Read the model definition and answer for the solid it produces. Units are mm, in the model's axes. A direction names the side the tool comes from. Give positions to 0.01 mm unless a question says otherwise; leave off trailing zeros. Loops run counter-clockwise (first coordinate to the right, second up) from the corner with the lowest first, then second, coordinate; pieces in that order, holes last. Notation, with made-up numbers: (60.5, 70) - (115.5, 70) arc R7 cw to (115.5, 82) - close; hole circle Ø11 at (-40, 17.5). An arc over 180 degrees is marked (long way). Write each question's results on one line, items separated by ' | '. Start each with the question number.
Q1. The part is cut by section B-B, the plane z = 0. Write down the section's boundary in (x, y).
Q2. Given pin 1 (3 mm diameter, centred on y = 5.5, z = 6, fed in from -X); pin 2 (2 mm diameter, centred on y = 13.5, z = -4.5, fed in from -X); pin 3 (4 mm diameter, centred on x = -31, y = 5.5, fed in from -Z), each flat-ended and moving along its own axis, determine where each tip first touches the part or whether it passes through.
Q3. The part is cut by section D-D, the plane x = -7.5. Write down the section's boundary in (y, z).
Q4. Find the intervals of material crossed by line 1 (X direction, y = 6, z = -6.75); line 2 (Z direction, x = -14.5, y = 2.75); line 3 (Y direction, x = -14, z = 1), in increasing order. Write a range as from..to.
Q5. For faces 1 (the flat face through (14, 17, 0)), 2 (the cylindrical face through (5.997, 13.451, -1.843)), determine the directions among +Z, -Z, +X, -X, +Y, -Y from which every point of the face is accessible in a straight line to the end or side of a thin tool.
Q6. The part is cut by section C-C, the plane y = 6.25. Write down the section's boundary in (x, z).
Q7. Determine the mould class of faces 3 (the cylindrical face through (-19.431, 4.93, 8.134)), 4 (the flat face through (-25, 5, 3)), 5 (the cylindrical face through (-35.35, 2.26, -0.61)) for opening direction Z: +Z half, -Z half, draft (parallel to the pull), parting line (faces both ways), or undercut.
Q8. The part is cut by section A-A, the plane z = 4.5. Write down the section's boundary in (x, y).
```python
from build123d import *

# Parameters (mm, degrees)
SKETCH_1_W      = 50
SKETCH_1_H      = 25
SKETCH_1_R      = 8.5
SKETCH_1_R_2    = 3
EXTRUDE_1_DEPTH = 10
SKETCH_2_R      = 2.808756841
EXTRUDE_2_DEPTH = 21
SKETCH_1_3_R    = 8.5
EXTRUDE_3_DEPTH = 17


with BuildPart() as part:
    # Sketch 1 → Extrude 1 (new body)
    # profile 1 of 2: a face of its own
    with BuildSketch(Plane(origin=(0, 0, 0), x_dir=(1, 0, 0), z_dir=(0, 1, 0))):
        Rectangle(SKETCH_1_W, SKETCH_1_H)
        with Locations((14.294554455, 0)):
            Circle(SKETCH_1_R, mode=Mode.SUBTRACT)
        with Locations(Location((-16.76980198, 6.75, 0), (0, 0, 270))):
            Circle(SKETCH_1_R_2, mode=Mode.SUBTRACT)
        with Locations(Location((-16.76980198, -6.75, 0), (0, 0, 270))):
            Circle(SKETCH_1_R_2, mode=Mode.SUBTRACT)
    # profile 2 of 2: a face of its own
    with BuildSketch(Plane(origin=(0, 0, 0), x_dir=(1, 0, 0), z_dir=(0, 1, 0))):
        with Locations((14.294554455, 0)):
            Circle(SKETCH_1_R)
    extrude(amount=EXTRUDE_1_DEPTH)

    # Sketch 2 → Extrude 2 (add)
    with BuildSketch(Plane.ZY.offset(25)):
        with Locations((0, 5)):
            Circle(SKETCH_2_R)
    extrude(amount=EXTRUDE_2_DEPTH)

    # Sketch 1_3 → Extrude 3 (add)
    with BuildSketch(Plane(origin=(0, 0, 0), x_dir=(1, 0, 0), z_dir=(0, 1, 0))):
        with Locations(Location((14.294554455, 0, 0), (0, 0, 270))):
            Circle(SKETCH_1_3_R)
    extrude(amount=EXTRUDE_3_DEPTH)


solid = part.part
```
Check sheet entries:
1) outline: (-46, 2.19) - (-25, 2.19) - (-25, 0) - (25, 0) - (25, 10) - (22.79, 10) - (22.79, 17) - (5.79, 17) - (5.79, 10) - (-25, 10) - (-25, 7.81) - (-46, 7.81) - close
2) pin 1: stops at x = -25 | pin 2: stops at x = 6.55 | pin 3: stops at z = -2.81
3) outline: (0, -12.5) - (10, -12.5) - (10, 12.5) - (0, 12.5) - close
4) line 1: x = -25..-19.77, -13.77..25 | line 2: z = -12.5..-8.71, -4.79..4.79, 8.71..12.5 | line 3: y = 0..10
5) face 1: +Z, -Z, +X, -X, +Y | face 2: +Y
6) outline: (-46, -2.52) - (-25, -2.52) - (-25, -12.5) - (25, -12.5) - (25, 12.5) - (-25, 12.5) - (-25, 2.52) - (-46, 2.52) - close; hole circle Ø6 at (-16.77, -6.75); hole circle Ø6 at (-16.77, 6.75)
7) face 3: undercut | face 4: draft | face 5: parting line
8) outline: (-25, 0) - (-18.75, 0) - (-18.75, 10) - (-25, 10) - close; (-14.79, 0) - (25, 0) - (25, 10) - (21.51, 10) - (21.51, 17) - (7.08, 17) - (7.08, 10) - (-14.79, 10) - close
